Source: three-view drawing plus pictorial views. Frame: mm from the lowest corner of the part. Round coordinates to 2 decimals unless told otherwise and drop trailing zeros. Write each loop counter-clockwise with the first axis right and the second up, starting at its lowest first coordinate (ties: lowest second). Pieces come first, ordered by that corner, then holes. Notation, with made-up numbers: (66, -12.75) - (118, -12.75) arc R19 ccw to (118, 21.25) - close; hole circle Ø10 at (0, 79). An arc over 180 degrees is marked (long way). Write each question's results on one line, items separated by ' | '.
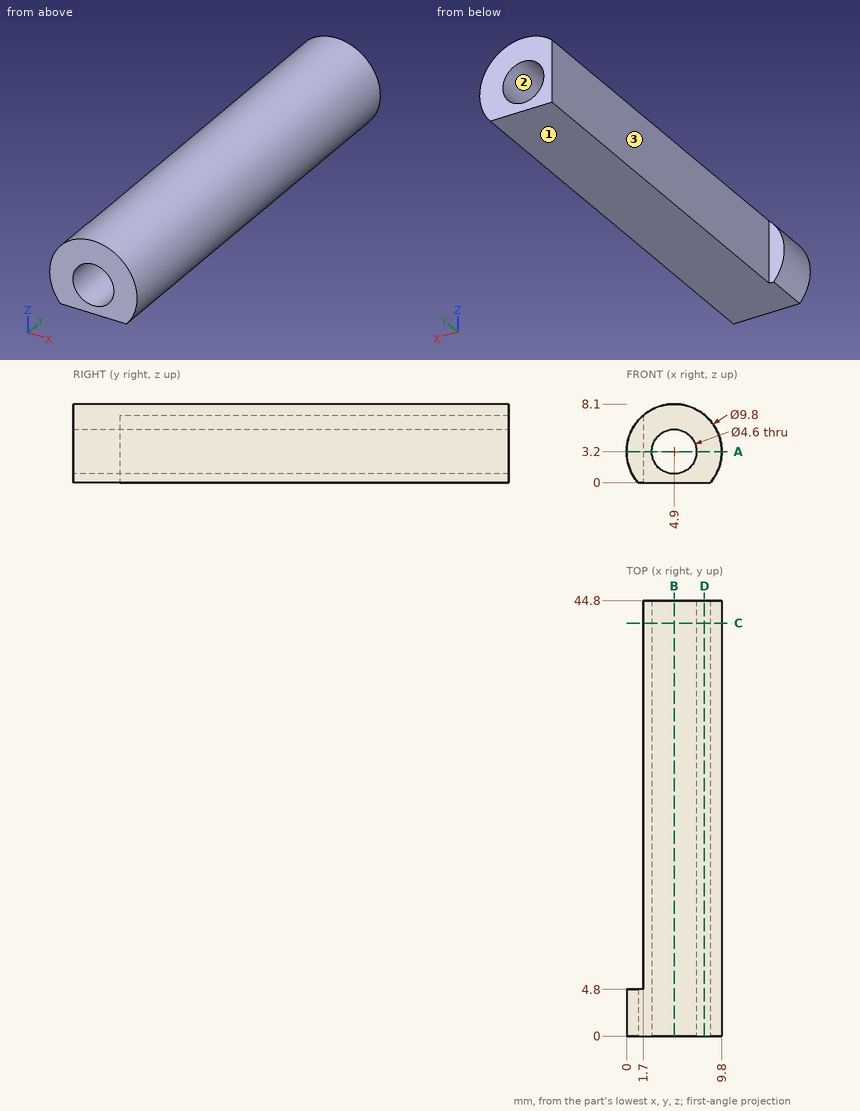
Q1. Section query D-D, the plane x = 8. Return loops of the section in (y, z), plus the area to 3 significant figures.
Answer block:
outline: (0, 0) - (44.8, 0) - (44.8, 6.99) - (0, 6.99) - close | area: 313 mm2
Q2. Section query B-B, the plane x = 4.9. Return loops of the section in (y, z).
Answer block:
outline: (0, 0) - (44.8, 0) - (44.8, 0.9) - (0, 0.9) - close; (0, 5.5) - (44.8, 5.5) - (44.8, 8.1) - (0, 8.1) - close
Q3. Pin query (flat end, axial travel): pin 1 (0.5 mm diameter, centred on x = 0.5, z = 4.5, fed in from +Y); pin 2 (2 mm diameter, centred on y = 27.5, z = 4.5, fed in from -X); pin 3 (1 mm diameter, centred on y = 30.5, z = 1, fed in from +X). Return the tip coordinate at first contact, or that it passes through.
Answer block:
pin 1: y = 4.8 | pin 2: x = 1.7 | pin 3: x = 9.5
Q4. Mould query, pull axis Z, two halves, no side actions, for the marked faces 1, 2 and 3. Classes: pulls with the +Z half, pulls with the -Z half, needs draft (parallel to the pull), parting line crosses it, or undercut.
Answer block:
face 1: pulls with the -Z half | face 2: undercut | face 3: needs draft
Q5. Section query A-A, the plane z = 3.2. Return loops of the section in (x, y).
Answer block:
outline: (0, 0) - (2.6, 0) - (2.6, 44.8) - (1.7, 44.8) - (1.7, 4.8) - (0, 4.8) - close; (7.2, 0) - (9.8, 0) - (9.8, 44.8) - (7.2, 44.8) - close
Q6. Ray query, line 1 along X through (y, z) = (13, 3); line 2 along Z through (x, y) = (4.75, 33.5); line 3 along X through (y, z) = (22, 2). Return the intervals inside material, ascending.
Answer block:
line 1: 1.7 to 2.61, 7.19 to 9.8 | line 2: 0 to 0.9, 5.5 to 8.1 | line 3: 1.7 to 2.94, 6.86 to 9.65
Q7. Section query C-C, the plane y = 42.5. Return loops of the section in (x, z).
Answer block:
outline: (1.7, 0) - (8.61, 0) arc R4.9 ccw to (1.7, 6.91) - close; hole circle Ø4.6 at (4.9, 3.2)
